Design review of the part built by this model. Coordinates are the model's own, in mm. Face numbers are marked on the shaded views. A direction names the side the tool comes from. Give positions to 0.01 mm unless a question says otherwise; leave off trailing zeros. Write each loop counter-clockwise with the first axis right and the second up, starting at its lowest first coordinate (ties: lowest second). Pieces come first, ordered by that corner, then holes.
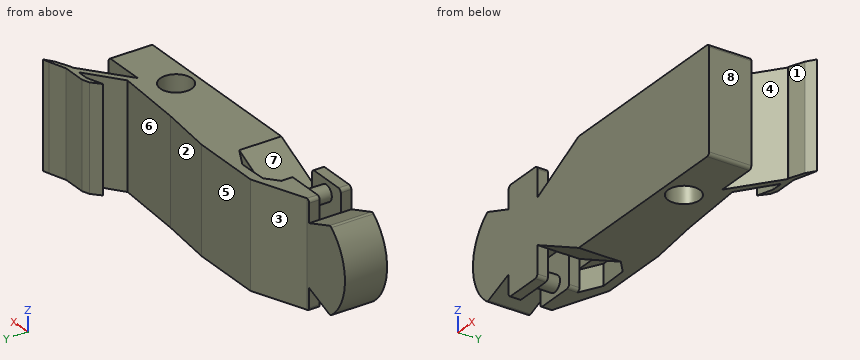
```python
from build123d import *

# Parameters (mm, degrees)
BOSS_EXTRUDE3_DEPTH = 101.6
SKETCH4_R           = 38.1
CUT_EXTRUDE1_DEPTH  = 508
CUT_EXTRUDE2_START  = -25.4
SKETCH16_W          = 101.6
SKETCH16_H          = 101.6
CUT_EXTRUDE2_DEPTH  = 50.8
SKETCH18_R          = 19.05
BOSS_EXTRUDE4_DEPTH = 50.8
CUT_EXTRUDE6_START  = -101.6
CUT_EXTRUDE6_DEPTH  = 101.6
FILLET2_R           = 7.62
BOSS_EXTRUDE7_DEPTH = 254
BOSS_EXTRUDE9_DEPTH = 254
CUT_EXTRUDE11_DEPTH = 50.8
CUT_EXTRUDE12_DEPTH = 50.8


with BuildPart() as part:
    # Sketch1 → Boss-Extrude3 (new body)
    with BuildSketch(Plane(origin=(0, 0, 0), x_dir=(1, 0, 0), z_dir=(0, 1, 0))):
        with BuildLine():
            ThreePointArc((-355.6, 127), (-482.6, 0), (-355.6, -127))
            Line((-355.6, -127), (355.6, -127))
            Line((355.6, -127), (355.6, 127))
            Line((355.6, 127), (-355.6, 127))
        make_face()
    extrude(amount=BOSS_EXTRUDE3_DEPTH)

    # Sketch4 → Cut-Extrude1 (cut)
    with BuildSketch(Plane.XY.offset(127)):
        with Locations((191.262, 50.8)):
            Circle(SKETCH4_R)
    extrude(amount=-CUT_EXTRUDE1_DEPTH, mode=Mode.SUBTRACT)

    # Sketch16 → Cut-Extrude2 (cut)
    with BuildSketch(Plane(origin=(0, 101.6, 0), x_dir=(1, 0, 0), z_dir=(0, 1, 0)).offset(CUT_EXTRUDE2_START)):
        with Locations((-304.8, 76.2)):
            Rectangle(SKETCH16_W, SKETCH16_H)
        with Locations((-304.8, -76.2)):
            Rectangle(SKETCH16_W, SKETCH16_H)
    extrude(amount=-CUT_EXTRUDE2_DEPTH, mode=Mode.SUBTRACT)

    # Sketch18 → Boss-Extrude4 (add)
    with BuildSketch(Plane(origin=(0, 25.4, 0), x_dir=(1, 0, 0), z_dir=(0, 1, 0))):
        with Locations(Location((-304.8, -95.885, 0), (0, 0, 270))):
            Circle(SKETCH18_R)
        with Locations(Location((-304.8, 95.885, 0), (0, 0, 90))):
            Circle(SKETCH18_R)
    extrude(amount=BOSS_EXTRUDE4_DEPTH)

    # Sketch23 → Cut-Extrude6 (cut)
    with BuildSketch(Plane(origin=(0, 101.6, 0), x_dir=(1, 0, 0), z_dir=(0, 1, 0)).offset(CUT_EXTRUDE6_START)):
        with BuildLine():
            Line((-355.6, -127), (-355.6, -73.963969071))
            Line((-355.6, -73.963969071), (-431.029237977, -102.173529146))
            ThreePointArc((-431.029237977, -102.173529146), (-395.304922859, -120.633822375), (-355.6, -127))
        make_face()
        Polygon((-254, -53.893344298), (-254, -127), (-107.585974166, -127), align=None)
        with BuildLine():
            Line((-355.6, 73.963969071), (-431.029237977, 102.173529146))
            ThreePointArc((-431.029237977, 102.173529146), (-395.304922859, 120.633822375), (-355.6, 127))
            Line((-355.6, 127), (-355.6, 73.963969071))
        make_face()
        Polygon((-254, 127), (-107.585974166, 127), (-254, 53.893344298), align=None)
    extrude(amount=CUT_EXTRUDE6_DEPTH, mode=Mode.SUBTRACT)

    # Fillet2
    fillet2_edges = [part.edges().sort_by_distance(p)[0] for p in [
        (-431.029237977, 50.8, -102.173529146),
        (-355.6, 12.7, -127),
        (-355.6, 12.7, 127),
        (-254, 12.7, -127),
        (-254, 88.9, -127),
        (-431.029237977, 50.8, 102.173529146),
        (-254, 88.9, 127),
        (-355.6, 88.9, -127),
        (-254, 12.7, 127),
        (355.6, 50.8, -127),
        (355.6, 50.8, 127),
        (-355.6, 88.9, 127),
    ]]
    fillet(fillet2_edges, radius=FILLET2_R)



with BuildPart() as body_2:
    # Sketch24 → Boss-Extrude7 (new body)
    with BuildSketch(Plane.XY.offset(127)):
        Polygon((362.058648087, 185.307634776), (252.61496451, 101.6), (225.581006965, 101.6), (338.66530168, 185.506014364), (334.087126159, 185.506014364), (309.686436817, 185.506014364), (271.381724032, 172.688112617), (292.121811526, 191.358212215), (309.686436817, 197.210410065), (365.827860262, 197.210410065), (407.553014944, 210.606867151), (422.496366485, 214.52949693), (401.536186127, 199.959729178), (365.827860262, 185.109255188), align=None)
    extrude(amount=-BOSS_EXTRUDE7_DEPTH)


with BuildPart() as part_1:
    add(part.part)

    add(body_2.part)  # Boss-Extrude9 merges body 2
    # Sketch24<8> → Boss-Extrude9 (add)
    with BuildSketch(Plane.XY.offset(127)):
        Polygon((-347.98, 101.6), (225.581006965, 101.6), (255.712540846, 123.956923399), (84.982041767, 135.949988054), (-45.964353963, 150.837955987), (-109.054165893, 150.837955987), (-220.445592276, 150.837955987), align=None)
    extrude(amount=-BOSS_EXTRUDE9_DEPTH)

    # Sketch26 → Cut-Extrude11 (cut)
    with BuildSketch(Plane.XY.offset(127)):
        Polygon((-261.62, 101.6), (-230.279041818, 127.879160506), (-159.925021307, 129.63026439), (-107.585974166, 101.6), align=None)
    extrude(amount=-CUT_EXTRUDE11_DEPTH, mode=Mode.SUBTRACT)

    # Sketch27 → Cut-Extrude12 (cut)
    with BuildSketch(Plane(origin=(0, 0, -127), x_dir=(-1, 0, 0), z_dir=(0, 0, -1))):
        Polygon((107.606718178, 101.590603269), (138.94767636, 127.869763774), (209.301696871, 129.620867658), (261.640744012, 101.590603269), align=None)
    extrude(amount=-CUT_EXTRUDE12_DEPTH, mode=Mode.SUBTRACT)


solid = part_1.part
```
(1) Consider section D-D, the plane x = -304.8. Give the boundary of the cut face in (y, z) (3 decimals).
Resolved:
outline: (0, -127) - (25.4, -127) - (25.4, -114.935) - (76.2, -114.935) - (76.2, -127) - (118.271, -127) - (118.271, 127) - (76.2, 127) - (76.2, 114.935) - (25.4, 114.935) - (25.4, 127) - (0, 127) - close; hole (25.4, -76.835) - (76.2, -76.835) - (76.2, -25.4) - (25.4, -25.4) - close; hole (25.4, 25.4) - (76.2, 25.4) - (76.2, 76.835) - (25.4, 76.835) - close
(2) To check wall thickness, follow L1, parallel to X at y = 83, z = 108.5; L2, parallel to X at y = 50, z = -3; L3, parallel to X at y = 65, z = -67. State the ranges of each line that lie inside material, in increasing order.
Resolved:
L1: x = -355.6 to -254, -144.64 to 170.9, 211.63 to 355.6
L2: x = -482.56 to 153.17, 229.35 to 355.6
L3: x = -463.49 to -355.6, -227.75 to 155.91, 226.62 to 355.6
(3) Tool access review of the marked faces 4, 5, 6, 7 and 8: name each direction out of +Z, -Z, +X, -X, +Y, -Y from which nothing blocks a thin tool from reaching the whole face with its end or side.
Resolved:
face 4: +Z, -Z, +X
face 5: +Z, -Z, -X, +Y
face 6: +Z, -Z, +Y
face 7: +Z, -Y
face 8: +Z, -Z, +X, -Y
(4) Consider section A-A, the plane y = 50.8. Give the boundary of the cut face in (x, z) (3 decimals).
Resolved:
outline: (-434.483, -99.531) arc R7.62 ccw to (-427.081, -100.697) - (-355.6, -73.964) - (-355.6, -25.4) - (-254, -25.4) - (-254, -53.893) - (-107.586, -127) - (153.162, -127) - (153.162, 127) - (-107.586, 127) - (-254, 53.893) - (-254, 25.4) - (-355.6, 25.4) - (-355.6, 73.964) - (-427.081, 100.697) arc R7.62 ccw to (-434.483, 99.531) arc R127 ccw to start; circle Ø38.1 at (-304.8, -95.885); circle Ø38.1 at (-304.8, 95.885); (229.362, -127) - (347.98, -127) arc R7.62 ccw to (355.6, -119.38) - (355.6, 119.38) arc R7.62 ccw to (347.98, 127) - (229.362, 127) - close
(5) Consider section C-C, the plane z = -34. Give the boundary of the cut face in (x, y), then the cut area to 3 significant figures.
Resolved:
outline: (-477.96, 0) - (355.6, 0) - (355.6, 101.6) - (252.61, 101.6) - (362.06, 185.31) - (365.83, 185.11) - (401.54, 199.96) - (422.5, 214.53) - (407.55, 210.61) - (365.83, 197.21) - (309.69, 197.21) - (292.12, 191.36) - (271.38, 172.69) - (309.69, 185.51) - (338.67, 185.51) - (255.71, 123.96) - (84.98, 135.95) - (-45.96, 150.84) - (-220.45, 150.84) - (-347.98, 101.6) - (-477.96, 101.6) - close; hole (-355.6, 25.4) - (-254, 25.4) - (-254, 76.2) - (-355.6, 76.2) - close; hole circle Ø76.2 at (191.26, 50.8)
area: 100,000 mm2
(6) Consider section B-B, the plane x = 322. Give the boundary of the cut face in (y, z).
Resolved:
outline: (0, -127) - (101.6, -127) - (101.6, 127) - (0, 127) - close; (154.67, -127) - (173.14, -127) - (173.14, 127) - (154.67, 127) - close; (185.51, -127) - (197.21, -127) - (197.21, 127) - (185.51, 127) - close
(7) Mouldability with a two-part tool opening along X and no side actions: class the marked faces 1, 2 and 3 as pulls with the +X half, pulls with the -X half, needs draft (parallel to the pull), parting line crosses it, or undercut.
Resolved:
face 1: pulls with the +X half
face 2: undercut
face 3: pulls with the -X half
(8) Clearance check with flat-ended pins moving along their axes: P1, Ø20.5, axis at y = 86, z = 79, coming from the +X side; P2, Ø3, axis at y = 128.5, z = -83.5, coming from the +X side; P3, Ø1.5, axis at y = 177, z = -51, coming from the +X side; P4, Ø12, axis at x = -374, z = -77.5, coming from the -Y side. State where each tip first meets the part, or that it passes through.
Resolved:
P1: stops at x = 355.6
P2: stops at x = 289.75
P3: stops at x = 352.18
P4: stops at y = 0
